```python
from build123d import *

# Parameters (mm, degrees)
SKETCH_1_W        = 111
SKETCH_1_H        = 61
SKETCH_1_W_2      = 107
SKETCH_1_H_2      = 57
EXTRUDE_1_DEPTH   = 10
SKETCH_3_W        = 111
SKETCH_3_H        = 61
EXTRUDE_1_2_DEPTH = 2


with BuildPart() as part:
    # 草圖1 → Extrude 1 (new body)
    with BuildSketch(Plane(origin=(0, 0, 0), x_dir=(1, 0, 0), z_dir=(0, 1, 0))):
        with Locations((53.5, 28.5)):
            Rectangle(SKETCH_1_W, SKETCH_1_H)
        with Locations((53.5, 28.5)):
            Rectangle(SKETCH_1_W_2, SKETCH_1_H_2, mode=Mode.SUBTRACT)
    extrude(amount=-EXTRUDE_1_DEPTH)

    # 草圖3 → Extrude 1 2 (add)
    with BuildSketch(Plane(origin=(0, -10, 0), x_dir=(-1, 0, 0), z_dir=(0, -1, 0))):
        with Locations((-53.5, 28.5)):
            Rectangle(SKETCH_3_W, SKETCH_3_H)
    extrude(amount=EXTRUDE_1_2_DEPTH)


solid = part.part
```
The model under review builds one solid part; all positions refer to its coordinate system, in mm. A direction names the side the tool comes from. Round coordinates to 2 decimals unless told otherwise and drop trailing zeros. Order: outer loops, then holes, each group sorted by start corner. A loop starts at its lowest first (then second) coordinate and runs counter-clockwise, first axis right, second up. Notation, with made-up numbers: (-39.5, 67) -> (-4.5, 67) arc R36 cw to (-4.5, 106) -> close; hole circle Ø1 at (75.5, 34.25). An arc over 180 degrees is marked (long way). Use a Markdown table: item, result.
Q1. Clearance check with a flat-ended pin moving along its axis: P1, Ø5, axis at x = 97, z = -18, coming from the +Y side. State where the tip first meets the part, or that it passes through.
Values:
| item | result |
|---|---|
| P1 | stops at y = -10 |
Q2. Mouldability with a two-part tool opening along Z and no side actions: class faces 1 (the flat face through (54, -6, 2)), 2 (the flat face through (0, -5, -28)), 3 (the flat face through (53, -5, -57)), 4 (the flat face through (37, 0, 1)) as +Z half, -Z half, draft (parallel to the pull), parting line (faces both ways), or undercut.
Values:
| item | result |
|---|---|
| face 1 | +Z half |
| face 2 | undercut |
| face 3 | undercut |
| face 4 | draft |
Q3. We need section A-A on y = -2. Write out the cut boundary in (x, z).
Values:
| item | result |
|---|---|
| outline | (-2, -59) -> (109, -59) -> (109, 2) -> (-2, 2) -> close; hole (0, -57) -> (107, -57) -> (107, 0) -> (0, 0) -> close |
Q4. We need section B-B on z = -36. Write out the cut boundary in (x, y), then the cut area to 3 significant figures.
Values:
| item | result |
|---|---|
| outline | (-2, -12) -> (109, -12) -> (109, 0) -> (107, 0) -> (107, -10) -> (0, -10) -> (0, 0) -> (-2, 0) -> close |
| area | 262 mm^2 |
Q5. Tool access review of faces 5 (the flat face through (54, -6, -59)), 6 (the flat face through (53, -5, 0)): name each direction out of +Z, -Z, +X, -X, +Y, -Y from which nothing blocks a thin tool from reaching the whole face with its end or side.
Values:
| item | result |
|---|---|
| face 5 | -Z, +X, -X, +Y, -Y |
| face 6 | +Y |
Q6. For line 1 (Z direction, x = 54, y = -8.25); line 2 (X direction, y = -3, z = -5.5); line 3 (Y direction, x = 46, z = -35.5), list the stretches that pass through material, from the lowest coordinate up.
Values:
| item | result |
|---|---|
| line 1 | z = -59 to -57, 0 to 2 |
| line 2 | x = -2 to 0, 107 to 109 |
| line 3 | y = -12 to -10 |
Q7. We need section C-C on x = 14.5. Write out the cut boundary in (y, z).
Values:
| item | result |
|---|---|
| outline | (-12, -59) -> (0, -59) -> (0, -57) -> (-10, -57) -> (-10, 0) -> (0, 0) -> (0, 2) -> (-12, 2) -> close |
